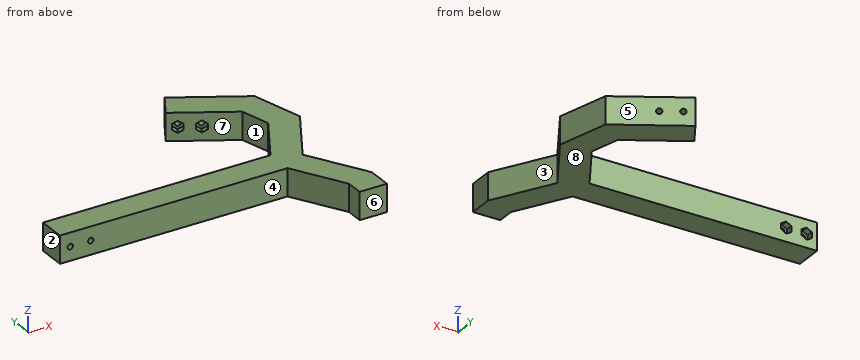
from build123d import *

# Parameters (mm, degrees)
SKETCH2_W          = 20
SKETCH2_H          = 20
SKETCH4_W          = 20
SKETCH4_H          = 20
CUT_EXTRUDE1_REACH = 228.27
SKETCH5_R          = 2
CUT_EXTRUDE2_START = -15
SKETCH5_3_R        = 2
CUT_EXTRUDE2_DEPTH = 5
CUT_EXTRUDE3_REACH = 204.251
SKETCH6_R          = 2
SKETCH6_5_R        = 2
CUT_EXTRUDE4_DEPTH = 5


with BuildPart() as part:
    # Sweep1: sweep along a path in Sketch1
    with BuildLine(Plane.XY) as sweep1_path:
        Line((0, 0), (44.828773608, -25.88190451))
        Line((44.828773608, -25.88190451), (52.676823753, -55.171226392))
        Line((52.676823753, -55.171226392), (26.794919243, -100))
        Line((26.794919243, -100), (52.676823753, -144.828773608))
        Line((52.676823753, -144.828773608), (52.676823753, -160))
    # Sketch2 → Sweep1 (sweep)
    with BuildSketch(Plane(origin=(0, 0, 0), x_dir=(0, 0, 1), z_dir=(-0.8660254037844382, 0.500000000000001, 0))):
        Rectangle(SKETCH2_W, SKETCH2_H)
    sweep(path=sweep1_path.line, transition=Transition.RIGHT)

    # Sweep3: sweep along a path in Sketch1<5>
    with BuildLine(Plane.XY) as sweep3_path:
        Line((26.794919243, -100), (-145.505080757, -100))
    # Sketch4 → Sweep3 (sweep)
    with BuildSketch(Plane(origin=(-145.505080757, -100, 0), x_dir=(0, 0, 1), z_dir=(-1, 0, 0))):
        Rectangle(SKETCH4_W, SKETCH4_H)
    sweep(path=sweep3_path.line)

    # Sketch5 → Cut-Extrude1 (cut, up to next)
    with BuildSketch(Plane(origin=(5, 8.660254038, 0), x_dir=(0.8660254037844382, -0.500000000000001, 0), z_dir=(0.500000000000001, 0.8660254037844382, 0)), mode=Mode.PRIVATE) as cut_extrude1_sk1:
        with Locations(Location((7.5, 0, 0), (0, 0, 180))):
            Circle(SKETCH5_R)
    cut_extrude1_tool1 = extrude(cut_extrude1_sk1.sketch, amount=-CUT_EXTRUDE1_REACH, mode=Mode.PRIVATE) & part.part
    # Sketch5 → Cut-Extrude1 (cut, up to next)
    with BuildSketch(Plane(origin=(5, 8.660254038, 0), x_dir=(0.8660254037844382, -0.500000000000001, 0), z_dir=(0.500000000000001, 0.8660254037844382, 0)), mode=Mode.PRIVATE) as cut_extrude1_sk2:
        with Locations(Location((22.5, 0, 0), (0, 0, 180))):
            Circle(SKETCH5_R)
    cut_extrude1_tool2 = extrude(cut_extrude1_sk2.sketch, amount=-CUT_EXTRUDE1_REACH, mode=Mode.PRIVATE) & part.part
    add(cut_extrude1_tool1.solids().sort_by_distance((11.495191, 4.910254, 0))[0], mode=Mode.SUBTRACT)
    add(cut_extrude1_tool2.solids().sort_by_distance((24.485572, -2.589746, 0))[0], mode=Mode.SUBTRACT)

    # Sketch5<3> → Cut-Extrude2 (cut)
    # profile 1 of 2: a face of its own
    with BuildSketch(Plane(origin=(5, 8.660254038, 0), x_dir=(0.8660254037844382, -0.500000000000001, 0), z_dir=(0.500000000000001, 0.8660254037844382, 0)).offset(CUT_EXTRUDE2_START)):
        Polygon((11.2, -2.136195996), (11.2, 2.136195996), (7.5, 4.272391992), (3.8, 2.136195996), (3.8, -2.136195996), (7.5, -4.272391992), align=None)
        with Locations(Location((7.5, 0, 0), (0, 0, 180))):
            Circle(SKETCH5_3_R, mode=Mode.SUBTRACT)
    # profile 2 of 2: a face of its own
    with BuildSketch(Plane(origin=(5, 8.660254038, 0), x_dir=(0.8660254037844382, -0.500000000000001, 0), z_dir=(0.500000000000001, 0.8660254037844382, 0)).offset(CUT_EXTRUDE2_START)):
        Polygon((26.2, -2.136195996), (26.2, 2.136195996), (22.5, 4.272391992), (18.8, 2.136195996), (18.8, -2.136195996), (22.5, -4.272391992), align=None)
        with Locations(Location((22.5, 0, 0), (0, 0, 180))):
            Circle(SKETCH5_3_R, mode=Mode.SUBTRACT)
    extrude(amount=-CUT_EXTRUDE2_DEPTH, mode=Mode.SUBTRACT)

    # Sketch6 → Cut-Extrude3 (cut, up to next)
    with BuildSketch(Plane(origin=(0, -90, -90), x_dir=(1, 0, 0), z_dir=(0, 1, 0)), mode=Mode.PRIVATE) as cut_extrude3_sk1:
        with Locations(Location((-138.005080757, -90, 0), (0, 0, 180))):
            Circle(SKETCH6_R)
    cut_extrude3_tool1 = extrude(cut_extrude3_sk1.sketch, amount=-CUT_EXTRUDE3_REACH, mode=Mode.PRIVATE) & part.part
    # Sketch6 → Cut-Extrude3 (cut, up to next)
    with BuildSketch(Plane(origin=(0, -90, -90), x_dir=(1, 0, 0), z_dir=(0, 1, 0)), mode=Mode.PRIVATE) as cut_extrude3_sk2:
        with Locations(Location((-123.005080757, -90, 0), (0, 0, 180))):
            Circle(SKETCH6_R)
    cut_extrude3_tool2 = extrude(cut_extrude3_sk2.sketch, amount=-CUT_EXTRUDE3_REACH, mode=Mode.PRIVATE) & part.part
    add(cut_extrude3_tool1.solids().sort_by_distance((-138.005081, -90, 0))[0], mode=Mode.SUBTRACT)
    add(cut_extrude3_tool2.solids().sort_by_distance((-123.005081, -90, 0))[0], mode=Mode.SUBTRACT)

    # Sketch6<5> → Cut-Extrude4 (cut)
    # profile 1 of 2: a face of its own
    with BuildSketch(Plane(origin=(0, -90, -90), x_dir=(1, 0, 0), z_dir=(0, 1, 0))):
        Polygon((-134.305080757, -92.136195996), (-134.305080757, -87.863804004), (-138.005080757, -85.727608008), (-141.705080757, -87.863804004), (-141.705080757, -92.136195996), (-138.005080757, -94.272391992), align=None)
        with Locations(Location((-138.005080757, -90, 0), (0, 0, 180))):
            Circle(SKETCH6_5_R, mode=Mode.SUBTRACT)
    # profile 2 of 2: a face of its own
    with BuildSketch(Plane(origin=(0, -90, -90), x_dir=(1, 0, 0), z_dir=(0, 1, 0))):
        Polygon((-119.305080757, -92.136195996), (-119.305080757, -87.863804004), (-123.005080757, -85.727608008), (-126.705080757, -87.863804004), (-126.705080757, -92.136195996), (-123.005080757, -94.272391992), align=None)
        with Locations(Location((-123.005080757, -90, 0), (0, 0, 180))):
            Circle(SKETCH6_5_R, mode=Mode.SUBTRACT)
    extrude(amount=-CUT_EXTRUDE4_DEPTH, mode=Mode.SUBTRACT)


solid = part.part
The listing builds one solid part. Answer for the finished solid, in the listing's coordinates (mm). Face numbers are marked on the shaded views. A direction names the side the tool comes from. Give positions to 0.01 mm unless a question says otherwise; leave off trailing zeros. Write each loop counter-clockwise with the first axis right and the second up, starting at its lowest first coordinate (ties: lowest second). Pieces come first, ordered by that corner, then holes. Notation, with made-up numbers: (44.5, -38) - (76.5, -38) arc R26 ccw to (76.5, -4) - close; hole circle Ø5 at (37, 36.25). An arc over 180 degrees is marked (long way). One line per question, with ' | ' between items. Start each with the question number.
1. Determine the mould class of the marked faces 6, 7 and 8 for opening direction Y: +Y half, -Y half, draft (parallel to the pull), parting line (faces both ways), or undercut.
2. Straight lines are drawn through the part: line 1 (Y direction, x = -131, z = 7); line 2 (Y direction, x = 24.5, z = 1.25); line 3 (Y direction, x = 33.5, z = 0.25). For each, find the intervals that lie inside material, in ascending order.
3. Section C-C, the plane y = -49 is taken. Determine the outline of the cut face in (x, z), then the cut area to 3 significant figures.
4. For the marked faces 1, 2, 3, 4 and 5, determine the directions among +Z, -Z, +X, -X, +Y, -Y from which every point of the face is accessible in a straight line to the end or side of a thin tool.
5. Section A-A, the plane z = 6.5 is taken. Determine the outline of the cut face in (x, y), then the cut area to 3 significant figures.
6. Given P1, Ø10, axis at y = -19.5, z = -2, coming from the -X side; P2, Ø9, axis at y = -151, z = -2.5, coming from the +X side; P3, Ø8, axis at y = -39, z = 4.5, coming from the +X side, each flat-ended and moving along its own axis, determine where each tip first touches the part or whether it passes through.
7. Section B-B, the plane x = -86.5 is taken. Determine the outline of the cut face in (y, z), then the cut area to 3 significant figures.
Result:
1) face 6: -Y half | face 7: undercut | face 8: draft
2) line 1: y = -110 to -90 | line 2: y = -116.03 to -83.97, -25.69 to -5.69 | line 3: y = -131.61 to -68.39, -30.89 to -7.79
3) outline: (40.67, -10) - (61.38, -10) - (61.38, 10) - (40.67, 10) - close | area: 414 mm2
4) face 1: +Z, -Z, -X | face 2: +Z, -Z, -X, +Y, -Y | face 3: +Z, -Z, +X | face 4: +Z, -Z, -X, -Y | face 5: +Z, -Z, +X, +Y
5) outline: (-145.51, -110) - (21.02, -110) - (42.68, -147.51) - (42.68, -160) - (62.68, -160) - (62.68, -142.15) - (38.34, -100) - (63.41, -56.58) - (53.42, -19.29) - (5, 8.66) - (-5, -8.66) - (36.24, -32.47) - (41.95, -53.76) - (21.02, -90) - (-145.51, -90) - close | area: 7,290 mm2
6) P1: stops at x = 5.11 | P2: stops at x = 62.68 | P3: stops at x = 59.77
7) outline: (-110, -10) - (-90, -10) - (-90, 10) - (-110, 10) - close | area: 400 mm2
